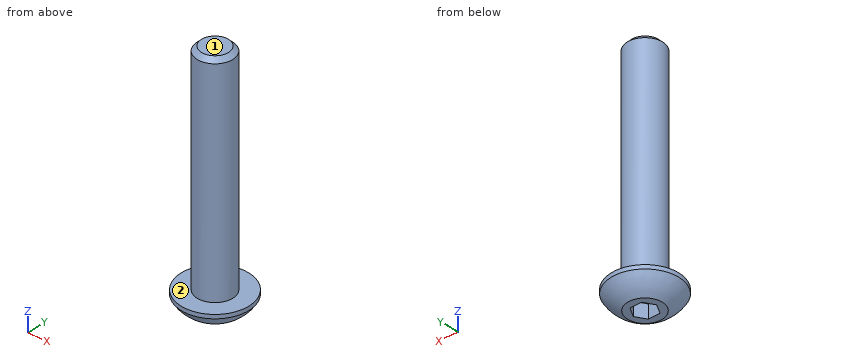
Autodesk Inventor part; units mm, degrees
ref_plane "YZ Plane" through (0, 0, 0) normal (1, 0, 0) x (0, 1, 0)
ref_plane "XZ Plane" through (0, 0, 0) normal (0, 1, 0) x (-1, 0, 0)
ref_plane "XY Plane" through (0, 0, 0) normal (0, 0, 1) x (1, 0, 0)
sketch "Sketch1" plane through (0, 0, 0) normal (0, 0, 1) x (1, 0, 0)
  circle A0 centre (0, 0) radius 2.0828
  dimension "d0" = 4.1656
extrude "Extrusion1" add sketch "Sketch1" along normal blind 25.4
sketch "Sketch2" plane through (0, 0, 0) normal (0, 1, 0) x (-1, 0, 0)
  line L0 (0, 0) -> (0, -2.2098)
  line L1 (0, 0) -> (3.9624, 0)
  line L2 (0, -2.2098) -> (2.032, -2.2098)
  line L3 (3.9624, 0) -> (3.9624, 3.6562) construction
  arc A0 (2.032, -2.2098) -> (3.9624, -0.4599) centre (0.1837, 1.7689) ccw
  line L4 (4.5847, 0.6553) -> (4.5847, -0.2608) construction
  line L5 (3.9624, -0.4599) -> (3.9624, 0)
  dimension "d3" = 2.2098
  dimension "d6" = 2.032
  dimension "d19" = 3.9624
revolve "Revolution1" add sketch "Sketch2" angle 360 about axis through (0, 0, 0) along (0, 0, -1)
sketch "Sketch3" plane through (0, 0, -2.2098) normal (0, 0, -1) x (-1, 0, 0)
  circle A0 centre (0, 0) radius 2.032
  line L0 (-0.6874, 1.1906) -> (0.6874, 1.1906)
  line L1 (0.6874, 1.1906) -> (1.3748, 0)
  line L2 (1.3748, 0) -> (0.6874, -1.1906)
  line L3 (0.6874, -1.1906) -> (-0.6874, -1.1906)
  line L4 (-0.6874, -1.1906) -> (-1.3748, 0)
  line L5 (-1.3748, 0) -> (-0.6874, 1.1906)
  dimension "d8" = 2.3813
extrude "Extrusion2" cut sketch "Sketch3" against normal blind 1.5875 contours L0 L1 L2 L3 L4 L5
chamfer "Chamfer1" distance 0.508 angle 45 1 edges at (-2.0828, 0, 25.4)
thread "Thread1"
properties part number "10-32 x500 button head" material "Steel"
Work out the finished part from the listing and answer in its coordinate system (mm). Face numbers are marked on the shaded views. A direction names the side the tool comes from. Round coordinates to 2 decimals unless told otherwise and drop trailing zeros. Order: outer loops, then holes, each group sorted by start corner. A loop starts at its lowest first (then second) coordinate and runs counter-clockwise, first axis right, second up. Notation, with made-up numbers: M 65.5,44 L 101.5,44 A17 cw 101.5,64 Z; hole C 20.5,82.5 d3. An arc over 180 degrees is marked long. Put each result on its own line as item: value. Start each with the question number.
Q1. Section A-A, the plane z = 4.5 is taken. Write down the section's boundary in (x, y).
Q2. A tool of negligible diameter and unlimited length cuts with its end or side. For the marked faces 1 and 2, from which of +Z, -Z, +X, -X, +Y, -Y can it reach the whole face along a straight path? Write none if from no direction.
Q3. Straight lines are drawn through the part: L1, parallel to Z at x = 2, y = -1.25; L2, parallel to Y at x = -1, z = 7.5; L3, parallel to X at y = -0.25, z = -0.5. For each, find the intervals that lie inside material, in ascending order. Write a range as [from, to].
Q4. Flat-ended cylindrical pins translate along their axes: pin 1 (0.7 mm diameter, centred on x = 0.5, y = 0.5, fed in from -Z); pin 2 (1 mm diameter, centred on y = 1.5, z = 20, fed in from +X); pin 3 (3 mm diameter, centred on y = 1, z = 6, fed in from +X). Find the tip coordinate at first contact, or state that the pin passes through.
Findings below:
1. outline: C 0,0 d4.17
2. face 1: +Z, +X, -X, +Y, -Y
2. face 2: +Z
3. L1: z = [-2.04, 0]
3. L2: y = [-1.83, 1.83]
3. L3: x = [-3.93, 3.93]
4. pin 1: stops at z = -0.62
4. pin 2: stops at x = 1.83
4. pin 3: stops at x = 2.08
